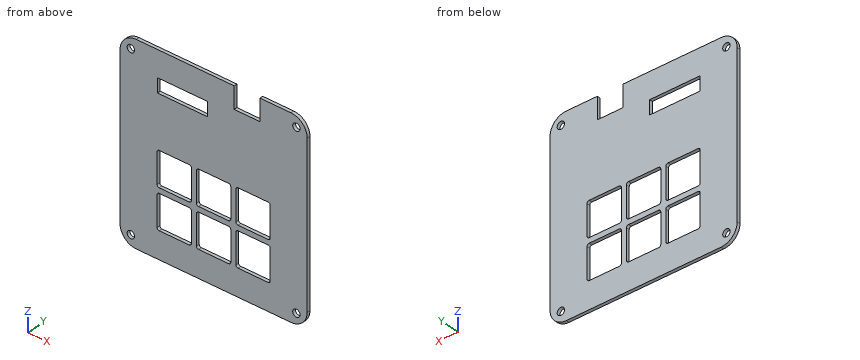
Autodesk Inventor part; units mm, degrees
ref_plane "YZ Plane" through (0, 0, 0) normal (1, 0, 0) x (0, 1, 0)
ref_plane "XZ Plane" through (0, 0, 0) normal (0, 1, 0) x (-1, 0, 0)
ref_plane "XY Plane" through (0, 0, 0) normal (0, 0, 1) x (1, 0, 0)
sketch "Sketch3" plane through (0, 0, 0) normal (0, 1, 0) x (-1, 0, 0)
  line L0 (-25.241, 1.984) -> (-11.271, 1.984)
  line L1 (-25.241, -13.891) -> (-11.271, -13.891)
  line L2 (-26.1935, 1.0315) -> (-26.1935, -12.9385)
  line L3 (-10.3185, 1.0315) -> (-10.3185, -12.9385)
  arc A0 (-25.241, 1.984) -> (-26.1935, 1.0315) centre (-25.241, 1.0315) ccw
  arc A1 (-10.3185, 1.0315) -> (-11.271, 1.984) centre (-11.271, 1.0315) ccw
  arc A2 (-26.1935, -12.9385) -> (-25.241, -13.891) centre (-25.241, -12.9385) ccw
  arc A3 (-11.271, -13.891) -> (-10.3185, -12.9385) centre (-11.271, -12.9385) ccw
  line L4 (-6.985, 1.984) -> (6.985, 1.984)
  line L5 (-6.985, -13.891) -> (6.985, -13.891)
  line L6 (-7.9375, 1.0315) -> (-7.9375, -12.9385)
  line L7 (7.9375, 1.0315) -> (7.9375, -12.9385)
  arc A4 (-6.985, 1.984) -> (-7.9375, 1.0315) centre (-6.985, 1.0315) ccw
  arc A5 (7.9375, 1.0315) -> (6.985, 1.984) centre (6.985, 1.0315) ccw
  arc A6 (-7.9375, -12.9385) -> (-6.985, -13.891) centre (-6.985, -12.9385) ccw
  arc A7 (6.985, -13.891) -> (7.9375, -12.9385) centre (6.985, -12.9385) ccw
  line L8 (11.271, 1.984) -> (25.241, 1.984)
  line L9 (11.271, -13.891) -> (25.241, -13.891)
  line L10 (10.3185, 1.0315) -> (10.3185, -12.9385)
  line L11 (26.1935, 1.0315) -> (26.1935, -12.9385)
  arc A8 (11.271, 1.984) -> (10.3185, 1.0315) centre (11.271, 1.0315) ccw
  arc A9 (26.1935, 1.0315) -> (25.241, 1.984) centre (25.241, 1.0315) ccw
  arc A10 (10.3185, -12.9385) -> (11.271, -13.891) centre (11.271, -12.9385) ccw
  arc A11 (25.241, -13.891) -> (26.1935, -12.9385) centre (25.241, -12.9385) ccw
  line L12 (-25.241, -16.272) -> (-11.271, -16.272)
  line L13 (-25.241, -32.147) -> (-11.271, -32.147)
  line L14 (-26.1935, -17.2245) -> (-26.1935, -31.1945)
  line L15 (-10.3185, -17.2245) -> (-10.3185, -31.1945)
  arc A12 (-25.241, -16.272) -> (-26.1935, -17.2245) centre (-25.241, -17.2245) ccw
  arc A13 (-10.3185, -17.2245) -> (-11.271, -16.272) centre (-11.271, -17.2245) ccw
  arc A14 (-26.1935, -31.1945) -> (-25.241, -32.147) centre (-25.241, -31.1945) ccw
  arc A15 (-11.271, -32.147) -> (-10.3185, -31.1945) centre (-11.271, -31.1945) ccw
  line L16 (-6.985, -16.272) -> (6.985, -16.272)
  line L17 (-6.985, -32.147) -> (6.985, -32.147)
  line L18 (-7.9375, -17.2245) -> (-7.9375, -31.1945)
  line L19 (7.9375, -17.2245) -> (7.9375, -31.1945)
  arc A16 (-6.985, -16.272) -> (-7.9375, -17.2245) centre (-6.985, -17.2245) ccw
  arc A17 (7.9375, -17.2245) -> (6.985, -16.272) centre (6.985, -17.2245) ccw
  arc A18 (-7.9375, -31.1945) -> (-6.985, -32.147) centre (-6.985, -31.1945) ccw
  arc A19 (6.985, -32.147) -> (7.9375, -31.1945) centre (6.985, -31.1945) ccw
  line L20 (11.271, -16.272) -> (25.241, -16.272)
  line L21 (11.271, -32.147) -> (25.241, -32.147)
  line L22 (10.3185, -17.2245) -> (10.3185, -31.1945)
  line L23 (26.1935, -17.2245) -> (26.1935, -31.1945)
  arc A20 (11.271, -16.272) -> (10.3185, -17.2245) centre (11.271, -17.2245) ccw
  arc A21 (26.1935, -17.2245) -> (25.241, -16.272) centre (25.241, -17.2245) ccw
  arc A22 (10.3185, -31.1945) -> (11.271, -32.147) centre (11.271, -31.1945) ccw
  arc A23 (25.241, -32.147) -> (26.1935, -31.1945) centre (25.241, -31.1945) ccw
  line L24 (-33.3375, -34.528) -> (33.3375, -34.528)
  line L25 (-33.3375, 34.528) -> (33.3375, 34.528)
  line L26 (-33.3375, -34.528) -> (-33.3375, 34.528)
  line L27 (33.3375, -34.528) -> (33.3375, 34.528)
  line L28 (-33.3375, 34.528) -> (-22.4409, 34.528) construction
  line L29 (-22.4409, 34.528) -> (-3.9497, 34.528)
  line L30 (-43.3375, -44.528) -> (43.3375, -44.528)
  line L31 (43.3375, -44.528) -> (43.3375, 44.528)
  line L32 (43.3375, 44.528) -> (-43.3375, 44.528)
  line L33 (-43.3375, 44.528) -> (-43.3375, -44.528)
  circle A24 centre (-38.3375, -39.528) radius 1.7
  circle A25 centre (38.3375, -39.528) radius 1.7
  circle A26 centre (-38.3375, 39.528) radius 1.7
  circle A27 centre (38.3375, 39.528) radius 1.7
  line L34 (-22.4409, 34.528) -> (-3.9409, 34.528)
  line L35 (-21.4315, 34.528) -> (-9.5255, 34.528)
  line L36 (-9.5255, 34.528) -> (-9.5255, 48.1303)
  line L37 (-9.5255, 48.1303) -> (-21.4315, 48.1303)
  line L38 (-21.4315, 48.1303) -> (-21.4315, 34.528)
  line L39 (2.7875, 26.028) -> (26.0375, 26.028)
  line L40 (26.0375, 26.028) -> (26.0375, 32.528)
  line L41 (26.0375, 32.528) -> (2.7875, 32.528)
  line L42 (2.7875, 32.528) -> (2.7875, 26.028)
  point P0 (0, 0)
  point P1 (-10.3185, -5.9535)
  point P2 (0, 0)
  point P3 (-21.4315, 44.528)
  point P4 (-9.5255, 44.528)
  point P5 (-9.5255, 34.528)
  dimension "d13" = 2.381
  dimension "d14" = 7.144
  dimension "d15" = 66.675
  dimension "d16" = 69.056
  dimension "d17" = 7.144
  dimension "d18" = 13.97
  dimension "d19" = 13.97
  dimension "d20" = 2.381
  dimension "d21" = 13.97
  dimension "d22" = 13.97
  dimension "d23" = 13.97
  dimension "d24" = 2.381
  dimension "d25" = 2.381
  dimension "d46" = 10
  dimension "d47" = 10
  dimension "d48" = 3.4
  dimension "d49" = 3.4
  dimension "d50" = 3.4
  dimension "d51" = 3.4
  dimension "d52" = 5
  dimension "d53" = 5
  dimension "d54" = 5
  dimension "d55" = 5
  dimension "d56" = 5
  dimension "d57" = 5
  dimension "d58" = 5
  dimension "d59" = 5
  dimension "d62" = 11.906
  dimension "d66" = 23.25
  dimension "d67" = 6.5
  dimension "d72" = 7.3
  dimension "d73" = 2
  dimension "d74" = 10
extrude "Extrusion4" add sketch "Sketch3" along normal blind 1.5 contours L26 L25 L27 L24 | L24 L27 L25 L36 L32 L31 L30 L33 L38 L26
fillet "Fillet4" radius 7.5 4 edges at (-43.3375, 0.75, -44.528) (-43.3375, 0.75, 44.528) (43.3375, 0.75, -44.528) (43.3375, 0.75, 44.528)
properties part number "case top"
Verification items for the finished model (mm, model axes). Round coordinates to 2 decimals unless told otherwise and drop trailing zeros. Loops run counter-clockwise (first coordinate to the right, second up) from the corner with the lowest first, then second, coordinate; pieces in that order, holes last. Notation, with made-up numbers: (89, 16.5) - (120, 16.5) arc R26 ccw to (120, 43.5) - close; hole circle Ø6 at (62, -26.75). An arc over 180 degrees is marked (long way). Use one line per item in the form item = value.
1. Section check A-A on x = 2. Record the cut outline in (y, z), and give its area (3 significant figures).
A:
outline = (0, -44.53) - (1.5, -44.53) - (1.5, -32.15) - (0, -32.15) - close; (0, -16.27) - (1.5, -16.27) - (1.5, -13.89) - (0, -13.89) - close; (0, 1.98) - (1.5, 1.98) - (1.5, 44.53) - (0, 44.53) - close
area = 86.0 mm²
2. Section check B-B on z = -23.5. Record the cut outline in (x, y), and give its area (3 significant figures).
A:
outline = (-43.34, 0) - (-26.19, 0) - (-26.19, 1.5) - (-43.34, 1.5) - close; (-10.32, 0) - (-7.94, 0) - (-7.94, 1.5) - (-10.32, 1.5) - close; (7.94, 0) - (10.32, 0) - (10.32, 1.5) - (7.94, 1.5) - close; (26.19, 0) - (43.34, 0) - (43.34, 1.5) - (26.19, 1.5) - close
area = 58.6 mm²
3. Section check C-C on x = -22. Record the cut outline in (y, z), and give its area (3 significant figures).
A:
outline = (0, -44.53) - (1.5, -44.53) - (1.5, -32.15) - (0, -32.15) - close; (0, -16.27) - (1.5, -16.27) - (1.5, -13.89) - (0, -13.89) - close; (0, 1.98) - (1.5, 1.98) - (1.5, 26.03) - (0, 26.03) - close; (0, 32.53) - (1.5, 32.53) - (1.5, 44.53) - (0, 44.53) - close
area = 76.2 mm²
4. Scan lines: probe 1 along X at (y, z) = (1.1, -31); probe 2 along Z at (x, y) = (12, 0.45); probe 3 along Z at (x, y) = (22.5, 0.3). Record each from-to range of solid material in increasing order.
A:
probe_1 = -43.34 to -26.19, -10.32 to -7.94, 7.94 to 10.32, 26.19 to 43.34
probe_2 = -44.53 to -32.15, -16.27 to -13.89, 1.98 to 34.53
probe_3 = -44.53 to -32.15, -16.27 to -13.89, 1.98 to 44.53
5. Section check D-D on x = 18.5. Record the cut outline in (y, z).
A:
outline = (0, -44.53) - (1.5, -44.53) - (1.5, -32.15) - (0, -32.15) - close; (0, -16.27) - (1.5, -16.27) - (1.5, -13.89) - (0, -13.89) - close; (0, 1.98) - (1.5, 1.98) - (1.5, 34.53) - (0, 34.53) - close
